Verification items for the finished model (mm, model axes). A direction names the side the tool comes from. Give positions to 0.01 mm unless a question says otherwise; leave off trailing zeros. Loops run counter-clockwise (first coordinate to the right, second up) from the corner with the lowest first, then second, coordinate; pieces in that order, holes last. Notation, with made-up numbers: (45, 68.5) - (89, 68.5) arc R4 ccw to (89, 73.5) - close; hole circle Ø1 at (54, 32.25). An arc over 180 degrees is marked (long way). Answer in a Markdown table with one row per item.
```python
from build123d import *

# Parameters (mm, degrees)
SKETCH1_R                = 41.275
SKETCH1_R_2              = 34.1503
EXTRUDE1_DEPTH           = 7.9248
CHAMFER1_SIZE            = 0.503174
CHAMFER2_SIZE            = 0.7747
CUT_EXTRUDE1_DEPTH       = 8.9248
FILLET1_R                = 0.4064
CIRPATTERN1_COUNT        = 4
FILLET1_OF_CIRPATTERN1_R = 0.4064


with BuildPart() as part:
    # Sketch1 → Extrude1 (new body)
    with BuildSketch(Plane.XY):
        Circle(SKETCH1_R)
        Circle(SKETCH1_R_2, mode=Mode.SUBTRACT)
    extrude(amount=EXTRUDE1_DEPTH)

    # Chamfer1
    chamfer1_edges = [part.edges().sort_by_distance(p)[0] for p in [
        (-41.275, 0, 0),
        (-41.275, 0, 7.9248),
    ]]
    chamfer(chamfer1_edges, length=CHAMFER1_SIZE)

    # Chamfer2
    chamfer2_edges = [part.edges().sort_by_distance(p)[0] for p in [
        (-34.1503, 0, 0),
        (-34.1503, 0, 7.9248),
    ]]
    chamfer(chamfer2_edges, length=CHAMFER2_SIZE)

    # Sketch2 → Cut-Extrude1 (cut, through all)
    with BuildSketch(Plane.XY.offset(7.9248)):
        with BuildLine():
            Line((26.854291633, 31.344419693), (25.07287509, 29.563003151))
            Line((25.07287509, 29.563003151), (29.563003151, 25.07287509))
            Line((29.563003151, 25.07287509), (31.344419693, 26.854291633))
            ThreePointArc((31.344419693, 26.854291633), (29.185832393, 29.185832393), (26.854291633, 31.344419693))
        make_face()
    cut_extrude1 = extrude(amount=-CUT_EXTRUDE1_DEPTH, mode=Mode.SUBTRACT)

    # Fillet1
    fillet1_edges = [part.edges().sort_by_distance(p)[0] for p in [
        (29.563003151, 25.07287509, 3.9624),
        (25.07287509, 29.563003151, 3.9624),
    ]]
    fillet(fillet1_edges, radius=FILLET1_R)

    # CirPattern1: Cut-Extrude1 ×4 about axis
    cirpattern1_axis = Axis((0, 0, 0), (0, 0, 1))
    for i in range(1, CIRPATTERN1_COUNT):
        add(cut_extrude1.rotate(cirpattern1_axis, i * 360 / CIRPATTERN1_COUNT), mode=Mode.SUBTRACT)

    # Fillet1 of CirPattern1
    fillet1_of_cirpattern1_edges = [part.edges().sort_by_distance(p)[0] for p in [
        (-25.07287509, 29.563003151, 3.9624),
        (-29.563003151, 25.07287509, 3.9624),
        (-29.563003151, -25.07287509, 3.9624),
        (-25.07287509, -29.563003151, 3.9624),
        (25.07287509, -29.563003151, 3.9624),
        (29.563003151, -25.07287509, 3.9624),
    ]]
    fillet(fillet1_of_cirpattern1_edges, radius=FILLET1_OF_CIRPATTERN1_R)


solid = part.part
```
Q1. Sectioned sample at A-A (z = 3.75). Record the cut outline in (x, y) (3 decimals).
Completed:
| item | result |
|---|---|
| outline | (-31.344, -26.854) - (-29.85, -25.36) arc R0.406 cw to (-29.276, -25.36) - (-25.36, -29.276) arc R0.406 cw to (-25.36, -29.85) - (-26.854, -31.344) arc R41.275 ccw to (26.854, -31.344) - (25.36, -29.85) arc R0.406 cw to (25.36, -29.276) - (29.276, -25.36) arc R0.406 cw to (29.85, -25.36) - (31.344, -26.854) arc R41.275 ccw to (31.344, 26.854) - (29.85, 25.36) arc R0.406 cw to (29.276, 25.36) - (25.36, 29.276) arc R0.406 cw to (25.36, 29.85) - (26.854, 31.344) arc R41.275 ccw to (-26.854, 31.344) - (-25.36, 29.85) arc R0.406 cw to (-25.36, 29.276) - (-29.276, 25.36) arc R0.406 cw to (-29.85, 25.36) - (-31.344, 26.854) arc R41.275 ccw to start; hole circle Ø68.301 at (0, 0) |
Q2. Draft check along Y on faces 1 (the face through (27.291, 27.345, 4.018)), 2 (the face through (12, 33, 7.925)), 3 (the face through (0.41, 40.91, 0.14)), 4 (the face through (40.91, -0.41, 0.14)). Enter one of: +Y half, -Y half, draft (parallel to the pull), parting line (faces both ways), or undercut.
Completed:
| item | result |
|---|---|
| face 1 | undercut |
| face 2 | draft |
| face 3 | +Y half |
| face 4 | parting line |
Q3. Thickness scan on line 1 (X direction, y = -25.5, z = 6.25); line 2 (Y direction, x = -26, z = 2.25); line 3 (X direction, y = -20.5, z = 4.5). Record the ranges inside material, lowest first.
Completed:
| item | result |
|---|---|
| line 1 | -32.46 to -29.99, -29.14 to -22.72, 22.72 to 29.14, 29.99 to 32.46 |
| line 2 | -32.06 to -30.49, -28.64 to -22.14, 22.14 to 28.64, 30.49 to 32.06 |
| line 3 | -35.82 to -27.31, 27.31 to 35.82 |
Q4. Sectioned sample at B-B (x = 0). Record the cut outline in (y, z) (3 decimals), and give its area (3 significant figures).
Completed:
| item | result |
|---|---|
| outline | (-41.275, 0.503) - (-40.772, 0) - (-34.925, 0) - (-34.15, 0.775) - (-34.15, 7.15) - (-34.925, 7.925) - (-40.772, 7.925) - (-41.275, 7.422) - close; (34.15, 0.775) - (34.925, 0) - (40.772, 0) - (41.275, 0.503) - (41.275, 7.422) - (40.772, 7.925) - (34.925, 7.925) - (34.15, 7.15) - close |
| area | 111 mm^2 |
Q5. Tool access check on faces 5 (the face through (-27.291, -27.345, 4.018)), 6 (the face through (-41.273, 0.409, 3.914)). Record the directions out of +Z, -Z, +X, -X, +Y, -Y that give a thin tool (end or side, any length) a straight path to the whole face; none if there is none.
Completed:
| item | result |
|---|---|
| face 5 | +Z, -Z |
| face 6 | +Z, -Z, -X |
Q6. Go/stop test with flat-tipped pins: P1, Ø1.5, axis at x = -14.5, z = 7, coming from the -Y side; P2, Ø3, axis at x = 8.5, z = 5.5, coming from the +Y side; P3, Ø2, axis at y = 1.5, z = 3.5, coming from the -X side. Record where each tip stops, or that it passes through.
Completed:
| item | result |
|---|---|
| P1 | y = -38.92 |
| P2 | y = 40.68 |
| P3 | x = -41.27 |
